Job drawing, mm, ordinate dimensions from the low corner. One solid piece. Give positions to 0.01 mm unless a question says otherwise; leave off trailing zeros. Loops run counter-clockwise (first coordinate to the right, second up) from the corner with the lowest first, then second, coordinate; pieces in that order, holes last.
Item 1: Saw through at A-A on x = 22. Give the cut face in (y, z) (1 decimal).
Item 2: Mould opens along Z. For the marked faces 1, 2 and 3 say: released by +Z, released by -Z, zero draft, split by the parting line, or undercut.
Item 3: Saw through at B-B on z = 20. Give the cut face in (x, y), plus the area to 3 significant figures.
Item 4: Saw through at D-D on y = 6.25. Give the number of separate pieces and of enclosed holes in the cut face.
Item 5: Probe probe 1 along X at (y, z) = (11.25, 32) (1 decimal); probe 2 along Z at (x, y) = (13, 19) (1 decimal). List the from-to ranges inside material, lowest first.
Item 6: Saw through at C-C on z = 32. Give the cut face in (x, y) (1 decimal), plus the area to 3 significant figures.
Item 7: Drop flat-ended pins along their axis: P1, Ø3, axis at x = 38, y = 20.5, coming from the +Z side (1 decimal); P2, Ø2, axis at x = 38, y = 6.5, coming from the +Z side (1 decimal); P3, Ø10, axis at x = 11.5, y = 23.5, coming from the -Z side. Give the stop position or say it passes through.
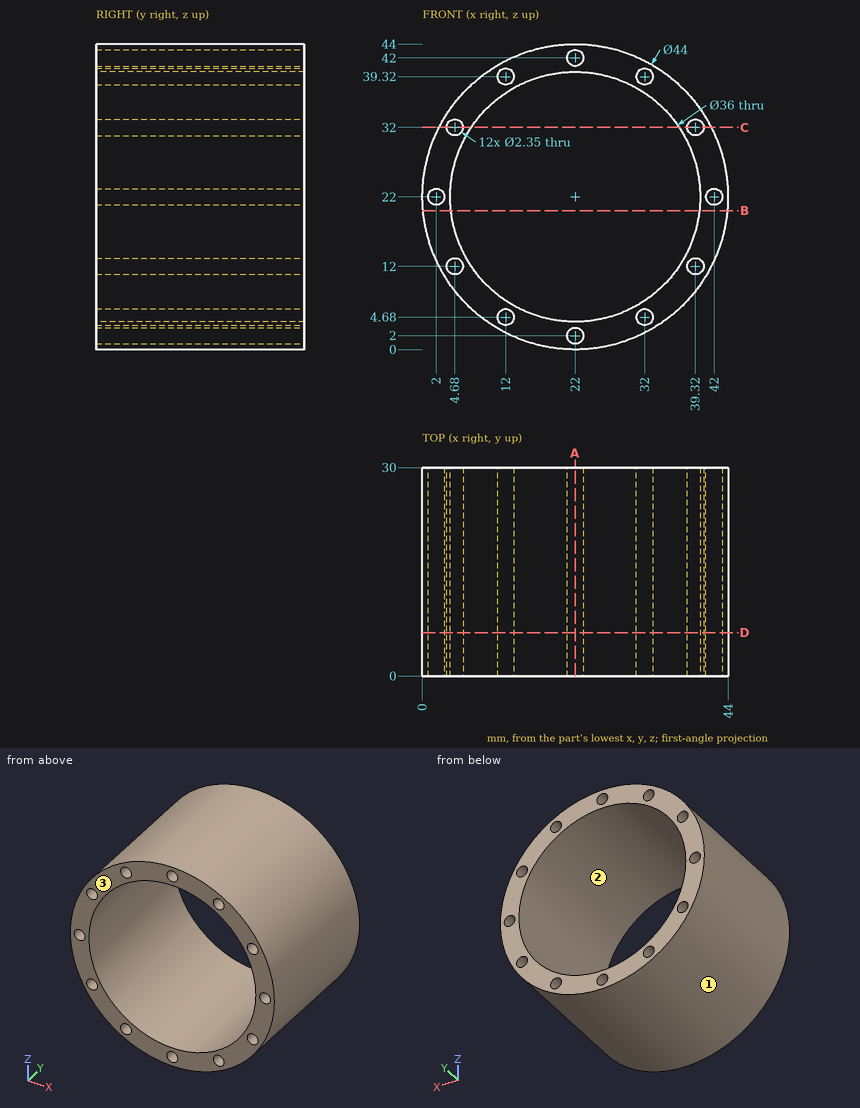
Results below:
1. outline: (0, 0) - (30, 0) - (30, 0.8) - (0, 0.8) - close; (0, 3.2) - (30, 3.2) - (30, 4) - (0, 4) - close; (0, 40) - (30, 40) - (30, 40.8) - (0, 40.8) - close; (0, 43.2) - (30, 43.2) - (30, 44) - (0, 44) - close
2. face 1: split by the parting line
2. face 2: undercut
2. face 3: zero draft
3. outline: (0.09, 0) - (4.11, 0) - (4.11, 30) - (0.09, 30) - close; (39.89, 0) - (43.91, 0) - (43.91, 30) - (39.89, 30) - close
3. area: 241 mm2
4. separate pieces: 1
4. enclosed holes: 13
5. probe 1: x = 2.4 to 3.5, 5.9 to 7, 37 to 38.1, 40.5 to 41.6
5. probe 2: z = 1.9 to 4.1, 5.3 to 6.4, 37.6 to 38.7, 39.9 to 42.1
6. outline: (2.4, 0) - (3.5, 0) - (3.5, 30) - (2.4, 30) - close; (5.9, 0) - (7, 0) - (7, 30) - (5.9, 30) - close; (37, 0) - (38.1, 0) - (38.1, 30) - (37, 30) - close; (40.5, 0) - (41.6, 0) - (41.6, 30) - (40.5, 30) - close
6. area: 137 mm2
7. P1: stops at z = 38.5
7. P2: stops at z = 38.1
7. P3: stops at z = 0.7
